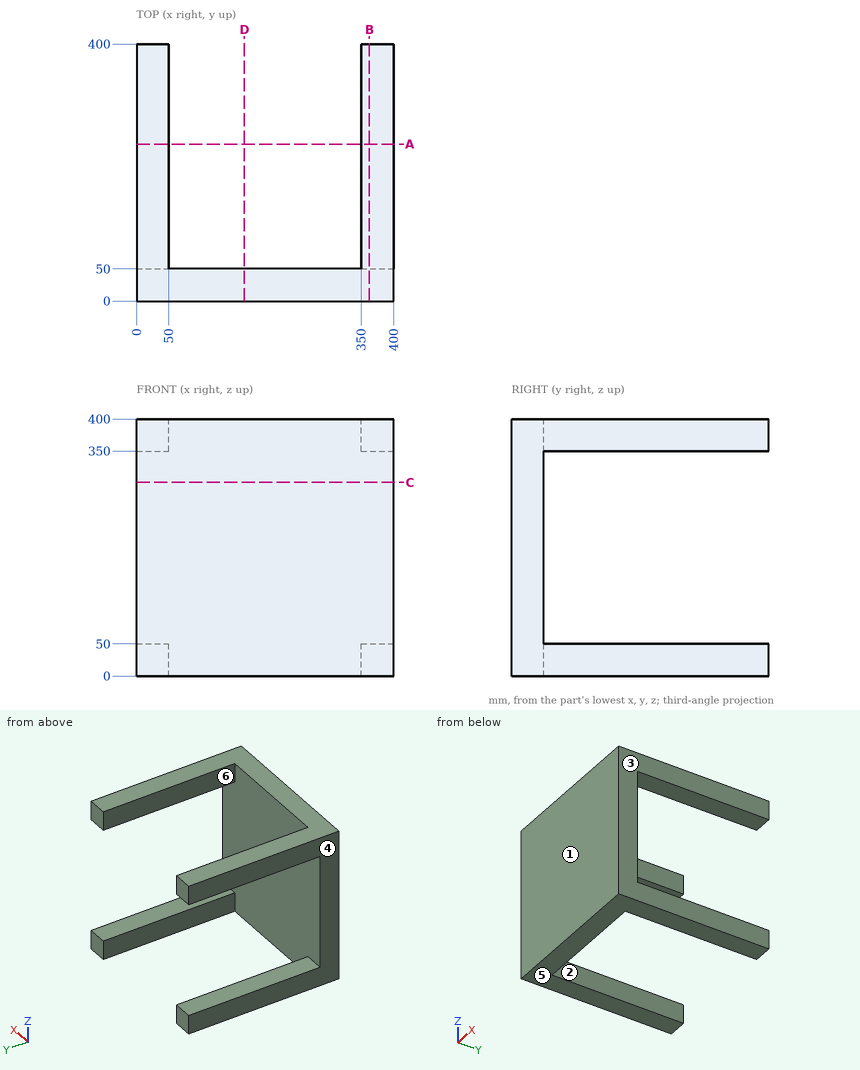
Input: dimensioned drawing with shaded views. Units: mm. Origin: part minimum x, y, z. A direction names the side the tool comes from. Give positions to 0.01 mm unless a question says otherwise; leave off trailing zeros. Write each loop counter-clockwise with the first axis right and the second up, starting at its lowest first coordinate (ties: lowest second). Pieces come first, ordered by that corner, then holes. Notation, with made-up numbers: M -33,18 L 5,18 A14 ccw 5,25 Z; hole C 8.5,5 d8. An arc over 180 degrees is marked long. Return JSON: item names as keys, results as strings. Group by question number.
1) Cut plane B-B, the plane x = 362.5. Output: boundary loops of the cut face in (y, z).
2) Material intervals for line 1 along Z through (x, y) = (379.5, 214); line 2 along Y through (x, z) = (229, 375), sorted ascending. Write a range as [from, to].
3) Cut plane D-D, the plane x = 168. Output: boundary loops of the cut face in (y, z).
4) Cut plane A-A, the plane y = 244. Output: boundary loops of the cut face in (x, z).
5) Pull-direction query (X, two-part tool) for the marked faces 1, 2, 3 and 4; classes: pulls with the +X half, pulls with the -X half, needs draft (parallel to the pull), parting line crosses it, or undercut.
6) Cut plane C-C, the plane z = 301.5. Output: boundary loops of the cut face in (x, y).
7) Pin query (flat end, axial travel): P1, Ø4, axis at x = 170.5, z = 259.5, coming from the +Y side. Return the tip coordinate at first contact, or that it passes through.
8) Set-up query: the marked faces 5 and 6. Return all of +Z, -Z, +X, -X, +Y, -Y with unobstructed straight access to the full face (end or side cutting, diameter ignored); none if empty.
Recorded:
{
 "1": {"outline": "M 0,0 L 400,0 L 400,50 L 50,50 L 50,350 L 400,350 L 400,400 L 0,400 Z"},
 "2": {"line 1": "z = [0, 50], [350, 400]", "line 2": "y = [0, 50]"},
 "3": {"outline": "M 0,0 L 50,0 L 50,400 L 0,400 Z"},
 "4": {"outline": "M 0,0 L 50,0 L 50,50 L 0,50 Z; M 0,350 L 50,350 L 50,400 L 0,400 Z; M 350,0 L 400,0 L 400,50 L 350,50 Z; M 350,350 L 400,350 L 400,400 L 350,400 Z"},
 "5": {"face 1": "needs draft", "face 2": "undercut", "face 3": "pulls with the +X half", "face 4": "pulls with the -X half"},
 "6": {"outline": "M 0,0 L 400,0 L 400,50 L 0,50 Z"},
 "7": {"P1": "stops at y = 50"},
 "8": {"face 5": "-Z, +X, -X, +Y, -Y", "face 6": "+Z, -Z, +Y"}
}
